Design review of the part built by this model. Coordinates are the model's own, in mm. Face numbers are marked on the shaded views. A direction names the side the tool comes from. Give positions to 0.01 mm unless a question says otherwise; leave off trailing zeros. Loops run counter-clockwise (first coordinate to the right, second up) from the corner with the lowest first, then second, coordinate; pieces in that order, holes last. Notation, with made-up numbers: (-4, 37) -> (20, 37) arc R17 ccw to (20, 53) -> close; hole circle Ø6 at (36.25, 46.5). An arc over 180 degrees is marked (long way). Answer as CSV lines item,"result".
Autodesk Inventor part; units mm, degrees
ref_plane "YZ Plane" through (0, 0, 0) normal (1, 0, 0) x (0, 1, 0)
ref_plane "XZ Plane" through (0, 0, 0) normal (0, 1, 0) x (-1, 0, 0)
ref_plane "XY Plane" through (0, 0, 0) normal (0, 0, 1) x (1, 0, 0)
sketch "Sketch1" plane through (0, 0, 0) normal (0, 0, 1) x (1, 0, 0)
  circle A0 centre (0, 0) radius 8
  dimension "d0" = 16
extrude "Extrusion1" add sketch "Sketch1" along normal blind 12
sketch "Sketch2" plane through (0, 0, 12) normal (0, 0, 1) x (1, 0, 0)
  circle A0 centre (0, 0) radius 5
  line L0 (1.9714, 4.5949) -> (4.9651, 0.5901)
  line L1 (4.9651, 0.5901) -> (2.9936, -4.0048)
  line L2 (2.9936, -4.0048) -> (-1.9714, -4.5949)
  line L3 (-1.9714, -4.5949) -> (-4.9651, -0.5901)
  line L4 (-4.9651, -0.5901) -> (-2.9936, 4.0048)
  line L5 (-2.9936, 4.0048) -> (1.9714, 4.5949)
  dimension "d3" = 10
extrude "Extrusion2" cut sketch "Sketch2" against normal blind 9 contours L1 L2 L3 L4 L5 L0
sketch "Sketch3" plane through (0, 0, 0) normal (0, 0, -1) x (-1, 0, 0)
  circle A0 centre (0, 0) radius 5
  dimension "d6" = 10
extrude "Extrusion3" add sketch "Sketch3" along normal blind 11
sketch "Sketch4" plane through (0, 0, -11) normal (0, 0, -1) x (-1, 0, 0)
  circle A0 centre (0, 0) radius 7
  dimension "d9" = 14
extrude "Extrusion4" add sketch "Sketch4" along normal blind 5
sketch "Sketch5" plane through (0, 0, -16) normal (0, 0, -1) x (-1, 0, 0)
  circle A0 centre (0, 0) radius 5
  dimension "d12" = 10
extrude "Extrusion5" add sketch "Sketch5" along normal blind 44
thread "Thread1"
chamfer "Chamfer1" distance 1 angle 45 1 edges at (-8, 0, 12)
equation "\"BendRadius\" = Thickness"
equation "\"BendReliefWidth\" = Thickness"
equation "\"BendReliefDepth\" = 0.5 * Thickness"
equation "\"CornerReliefSize\" = 4 * Thickness"
equation "\"MinimumRemnant\" = 2 * Thickness"
equation "\"TransitionRadius\" = BendRadius"
equation "\"JacobiRadiusSize\" = BendRadius"
equation "\"GapSize\" = Thickness"
properties part number "Adjusting Screw"
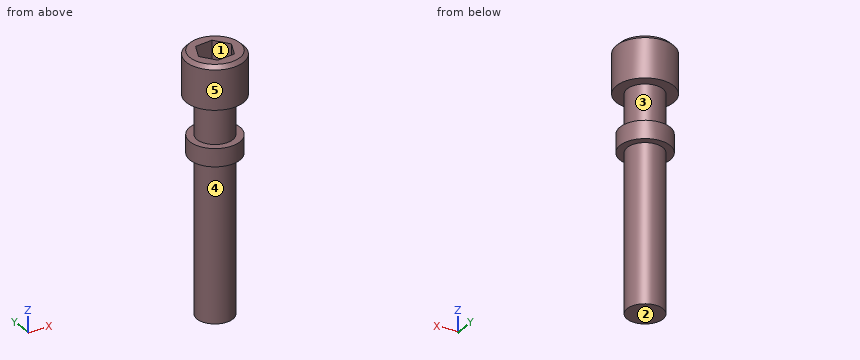
Q1. To check wall thickness, follow probe 1 along Z at (x, y) = (-5.5, 0); probe 2 along Y at (x, z) = (4, -42); probe 3 along Z at (x, y) = (-3.75, -1.25). State the ranges of each line that lie inside material, in increasing order. Write a range as from..to.
Filled sheet:
probe 1,"z = -16..-11, 0..12"
probe 2,"y = -3..3"
probe 3,"z = -60..3"
Q2. We need section C-C, the plane z = -13.5. State the section outline as (x, y) points, and give its area (3 significant figures).
Filled sheet:
outline,"circle Ø14 at (0, 0)"
area,"154 mm^2"
Q3. Clearance check with flat-ended pins moving along their axes: pin 1 Ø6 at (y, z) = (0, -34.5) entering from -X; pin 2 Ø6 at (x, z) = (5, -1) entering from -Y; pin 3 Ø4 at (x, z) = (4, -3.5) entering from -Y. State where each tip first meets the part, or that it passes through.
Filled sheet:
pin 1,"stops at x = -5"
pin 2,"stops at y = -7.7"
pin 3,"stops at y = -4.58"
Q4. We need section A-A, the plane x = 0. State the section outline as (y, z) points.
Filled sheet:
outline,"(-8, 0) -> (-5, 0) -> (-5, -11) -> (-7, -11) -> (-7, -16) -> (-5, -16) -> (-5, -60) -> (5, -60) -> (5, -16) -> (7, -16) -> (7, -11) -> (5, -11) -> (5, 0) -> (8, 0) -> (8, 11) -> (7, 12) -> (4.36, 12) -> (4.36, 3) -> (-4.36, 3) -> (-4.36, 12) -> (-7, 12) -> (-8, 11) -> close"
Q5. The part is to be moulded in two halves that separate along Z. For the marked faces 1, 2 and 3, say which applies: pulls with the +Z half, pulls with the -Z half, needs draft (parallel to the pull), parting line crosses it, or undercut.
Filled sheet:
face 1,"needs draft"
face 2,"pulls with the -Z half"
face 3,"undercut"
Q6. For the marked faces 4 and 5, list the 3-axis set-ups (+Z, -Z, +X, -X, +Y, -Y) from which the entire face can be reached by the end or side of a thin tool; tool diameter is ignored.
Filled sheet:
face 4,"-Z"
face 5,"+Z, -Z"
Q7. We need section B-B, the plane z = -36.5. State the section outline as (x, y) points, and give its area (3 significant figures).
Filled sheet:
outline,"circle Ø10 at (0, 0)"
area,"78.5 mm^2"
